from build123d import *

# Parameters (mm, degrees)
F1_DEPTH = 10
F3_DEPTH = 20
F4_R     = 10
F5_DEPTH = 30.001
F7_DEPTH = 5


with BuildPart() as f1:
    # F0 (on Top) → F1 (new body)
    with BuildSketch(Plane.XY):
        with BuildLine():
            Line((55, 20), (0, 20))
            ThreePointArc((0, 20), (-20, 0), (0, -20))
            Line((0, -20), (55, -20))
            ThreePointArc((55, -20), (75, 0), (55, 20))
        make_face()
    extrude(amount=F1_DEPTH)

    # F2 (on face) → F3 (join)
    with BuildSketch(Plane.XY.offset(10)):
        with BuildLine():
            ThreePointArc((2.4982464904, -20), (15.1095079365, -13.3395654143), (20.1554269498, 0))
            ThreePointArc((20.1554269498, 0), (15.1095079365, 13.3395654143), (2.4982464904, 20))
            Line((2.4982464904, 20), (0, 20))
            ThreePointArc((0, 20), (-20, 0), (0, -20))
            Line((0, -20), (2.4982464904, -20))
        make_face()
    extrude(amount=F3_DEPTH)

    # F4 (on face) → F5 (cut, through all)
    with BuildSketch(Plane.XY.offset(30)):
        Circle(F4_R)
    extrude(amount=-F5_DEPTH, mode=Mode.SUBTRACT)

    # F6 (on face) → F7 (cut)
    with BuildSketch(Plane.XY.offset(30)):
        with BuildLine():
            Line((-6.6143782777, 7.5), (-18.5404962177, 7.5))
            ThreePointArc((-18.5404962177, 7.5), (-20, 0), (-18.5404962177, -7.5))
            Line((-18.5404962177, -7.5), (-6.6143782777, -7.5))
            ThreePointArc((-6.6143782777, -7.5), (-10, 0), (-6.6143782777, 7.5))
        make_face()
        with BuildLine():
            Line((18.708052692, 7.5), (6.6143782777, 7.5))
            ThreePointArc((6.6143782777, 7.5), (9.1143782777, 4.1143782777), (10, 0))
            ThreePointArc((10, 0), (9.1143782777, -4.1143782777), (6.6143782777, -7.5))
            Line((6.6143782777, -7.5), (18.708052692, -7.5))
            ThreePointArc((18.708052692, -7.5), (20.1554269498, 0), (18.708052692, 7.5))
        make_face()
    extrude(amount=-F7_DEPTH, mode=Mode.SUBTRACT)


solid = f1.part
Could you check a few things on this model? Use its own coordinates, in mm. A direction names the side the tool comes from. Coordinates: 2 decimals unless noted, no trailing zeros. Loops run counter-clockwise (first coordinate to the right, second up) from the corner with the lowest first, then second, coordinate; pieces in that order, holes last.
1. For P1, Ø8, axis at x = 36, y = 7.5, coming from the +Z side; P2, Ø4, axis at x = 14, z = 26.5, coming from the -Y side; P3, Ø1.5, axis at x = -13, z = 27, coming from the +Y side; P4, Ø6, axis at x = 31.5, y = 14.5, coming from the -Z side, each with a flat end and sliding along its axis, tell me the tip position at first contact or that it passes through.
2. Imagine slicing it at D-D (z = 3.75). Please give me the cut outline in (x, y).
3. Imagine slicing it at A-A (z = 28). Please give me the cut outline in (x, y).
4. Imagine slicing it at B-B (x = -7.5). Please give me the cut outline in (y, z).
5. I need wall thicknesses on L1, parallel to Y at x = 0, z = 21.25; L2, parallel to X at y = 0, z = 13.5; L3, parallel to Z at x = 55.5, y = 1. Which ranges of each line are inside material? Lowest first, please.
6. We'd pull the mould along Y, two halves only. Please class faces 1 (the face through (27, 0, 0)), 2 (the face through (-20, 0, 15)), 3 (the face through (13, 7.5, 28)), 4 (the face through (26, 20, 7)): released by +Y, released by -Y, zero draft, split by the parting line, or undercut.
7. Imagine slicing it at C-C (y = 3). Please give me the cut outline in (x, z).
8. For faces 5 (the face through (-15, 0, 25)), 6 (the face through (0, -12, 30)), which set-ups out of +Z, -Z, +X, -X, +Y, -Y let a thin tool reach every point of the face, with its end or its side?
Computed values:
1. P1: stops at z = 10
1. P2: stops at y = -16.19
1. P3: stops at y = 15.81
1. P4: stops at z = 0
2. outline: (0, -20) - (55, -20) arc R20 ccw to (55, 20) - (0, 20) arc R20 ccw to start; hole circle Ø20 at (0, 0)
3. outline: (-18.54, -7.5) arc R20 ccw to (0, -20) - (2.5, -20) arc R20.16 ccw to (18.71, -7.5) - (6.61, -7.5) arc R10 cw to (-6.61, -7.5) - close; (-18.54, 7.5) - (-6.61, 7.5) arc R10 cw to (6.61, 7.5) - (18.71, 7.5) arc R20.16 ccw to (2.5, 20) - (0, 20) arc R20 ccw to start
4. outline: (-18.54, 0) - (-6.61, 0) - (-6.61, 25) - (-7.5, 25) - (-7.5, 30) - (-18.54, 30) - close; (6.61, 0) - (18.54, 0) - (18.54, 30) - (7.5, 30) - (7.5, 25) - (6.61, 25) - close
5. L1: y = -20 to -10, 10 to 20
5. L2: x = -20 to -10, 10 to 20.16
5. L3: z = 0 to 10
6. face 1: zero draft
6. face 2: split by the parting line
6. face 3: undercut
6. face 4: released by +Y
7. outline: (-19.77, 0) - (-9.54, 0) - (-9.54, 25) - (-19.77, 25) - close; (9.54, 0) - (74.77, 0) - (74.77, 10) - (19.93, 10) - (19.93, 25) - (9.54, 25) - close
8. face 5: +Z, +X, -X
8. face 6: +Z, +X, -X, +Y, -Y
